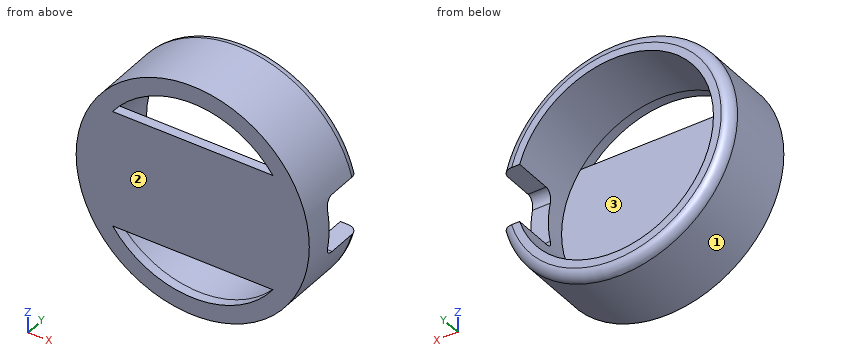
```python
from build123d import *

# Parameters (mm, degrees)
SKETCH1_R           = 6
SKETCH1_R_2         = 5.1
BOSS_EXTRUDE1_DEPTH = 3.5
SKETCH4_R           = 6
BOSS_EXTRUDE2_DEPTH = 0.5
SKETCH5_W           = 6
SKETCH5_H           = 3
CUT_EXTRUDE3_DEPTH  = 2.5
CUT_EXTRUDE4_DEPTH  = 1.5
FILLET1_R           = 0.5


with BuildPart() as part:
    # Sketch1 → Boss-Extrude1 (new body)
    with BuildSketch(Plane(origin=(0, 0, 0), x_dir=(1, 0, 0), z_dir=(0, 1, 0))):
        Circle(SKETCH1_R)
        Circle(SKETCH1_R_2, mode=Mode.SUBTRACT)
    extrude(amount=BOSS_EXTRUDE1_DEPTH)

    # Sketch4 → Boss-Extrude2 (add)
    with BuildSketch(Plane.XZ):
        Circle(SKETCH4_R)
    extrude(amount=BOSS_EXTRUDE2_DEPTH)

    # Sketch5 → Cut-Extrude3 (cut)
    with BuildSketch(Plane.XZ.offset(-3.5)):
        with Locations((3, 0)):
            Rectangle(SKETCH5_W, SKETCH5_H)
    extrude(amount=CUT_EXTRUDE3_DEPTH, mode=Mode.SUBTRACT)

    # Sketch7 → Cut-Extrude4 (cut, through all)
    with BuildSketch(Plane(origin=(0, 0, 0), x_dir=(1, 0, 0), z_dir=(0, 1, 0))):
        with BuildLine():
            Line((4.124318125, -3), (-4.124318125, -3))
            ThreePointArc((-4.124318125, -3), (0, -5.1), (4.124318125, -3))
        make_face()
        with BuildLine():
            Line((4.124318125, 3), (-4.124318125, 3))
            ThreePointArc((-4.124318125, 3), (0, 5.1), (4.124318125, 3))
        make_face()
    extrude(amount=-CUT_EXTRUDE4_DEPTH, mode=Mode.SUBTRACT)

    # Fillet1
    fillet1_edges = [part.edges().sort_by_distance(p)[0] for p in [
        (-6, 3.5, 0),
        (5.341949031, 1, -1.5),
        (5.341949031, 1, 1.5),
    ]]
    fillet(fillet1_edges, radius=FILLET1_R)


solid = part.part
```
Input: part model. Units: mm. Frame: model coordinates. Face numbers are marked on the shaded views. Coordinates: 2 decimals unless noted, no trailing zeros. Write each loop counter-clockwise with the first axis right and the second up, starting at its lowest first coordinate (ties: lowest second). Pieces come first, ordered by that corner, then holes. Notation, with made-up numbers: M 41,11 L 58,11 A23 cw 58,33 Z; hole C 61.25,5.5 d4. An arc over 180 degrees is marked long. Use one line per item in the form item = value.
Q1. Draft query along X for the marked faces 1, 2 and 3. Return one class per face: released by +X, released by -X, zero draft, split by the parting line, or undercut.
Answer below:
face_1 = split by the parting line
face_2 = zero draft
face_3 = undercut
Q2. Section B-B (y = -0.2). Return loops of the section in (x, z).
Answer below:
outline = C 0,0 d12; hole M -4.12,-3 A5.1 ccw 4.12,-3 Z; hole M -4.12,3 L 4.12,3 A5.1 ccw Z
Q3. Section A-A (x = 0). Return loops of the section in (y, z).
Answer below:
outline = M -0.5,-6 L 3,-6 A0.5 ccw 3.5,-5.5 L 3.5,-5.1 L -0.5,-5.1 Z; M -0.5,-3 L 0,-3 L 0,3 L -0.5,3 Z; M -0.5,5.1 L 3.5,5.1 L 3.5,5.5 A0.5 ccw 3,6 L -0.5,6 Z
Q4. Material intervals for probe 1 along Z at (x, y) = (0, 0.75); probe 2 along Y at (x, z) = (-4, -0.5); probe 3 along X at (y, z) = (1.6, 0), sorted ascending. Write a range as from..to.
Answer below:
probe_1 = -6..-5.1, 5.1..6
probe_2 = -0.5..0
probe_3 = -6..-5.1
Q5. First-contact query: pin 1 (1 mm diameter, centred on y = 2.5, z = -5, fed in from +X); pin 2 (1.1 mm diameter, centred on x = 5.5, z = 0, fed in from +Y); pin 3 (3 mm diameter, centred on x = 0, z = -1.5, fed in from +Y). Flat tips, straight axial feed; report the tip coordinate or a pass-through.
Answer below:
pin_1 = 3.97
pin_2 = 1
pin_3 = 0
Q6. Section C-C (z = 0). Return loops of the section in (x, y), plus the area to 4 significant figures.
Answer below:
outline = M -6,-0.5 L 6,-0.5 L 6,1 L 5.1,1 L 5.1,0 L -5.1,0 L -5.1,3.5 L -5.5,3.5 A0.5 ccw -6,3 Z
area = 10.00 mm²
Q7. Section D-D (y = 1.8). Return loops of the section in (x, z).
Answer below:
outline = M 4.87,-1.5 A5.1 cw long 4.87,1.5 L 5.81,1.5 A6 ccw long 5.81,-1.5 Z
